```python
from build123d import *

# Parameters (mm, degrees)
SKETCH1_R           = 1.25
SKETCH1_R_2         = 1.5875
SKETCH1_R_3         = 1.587499999
SKETCH1_R_4         = 3
BOSS_EXTRUDE1_DEPTH = 3.175


with BuildPart() as part:
    # Sketch1 → Boss-Extrude1 (new body)
    with BuildSketch(Plane(origin=(0, 0, 0), x_dir=(1, 0, 0), z_dir=(0, 1, 0))):
        with BuildLine():
            Line((-19.061691445, 152.305177286), (-29.109279467, 70.814859111))
            ThreePointArc((-29.109279467, 70.814859111), (-29.106764186, 70.406916612), (-29.000369251, 70.01308476))
            Line((-29.000369251, 70.01308476), (-24.900498144, 60.115120329))
            ThreePointArc((-24.900498144, 60.115120329), (-24.059191565, 59.263489811), (-22.862282328, 59.241590515))
            ThreePointArc((-22.862282328, 59.241590515), (0, 63.5), (22.862282328, 59.241590515))
            ThreePointArc((22.862282328, 59.241590515), (24.059191565, 59.263489811), (24.900498144, 60.115120329))
            Line((24.900498144, 60.115120329), (29.000369251, 70.01308476))
            ThreePointArc((29.000369251, 70.01308476), (29.106764186, 70.406916612), (29.109279467, 70.814859111))
            Line((29.109279467, 70.814859111), (19.061691445, 152.305177286))
            ThreePointArc((19.061691445, 152.305177286), (19.052985039, 152.398309253), (19.049778848, 152.491792328))
            ThreePointArc((19.049778848, 152.491792328), (0, 171.45), (-19.049778848, 152.491792328))
            ThreePointArc((-19.049778848, 152.491792328), (-19.052985039, 152.398309253), (-19.061691445, 152.305177286))
        make_face()
        with Locations(Location((-10.606601718, 163.006601718, 0), (0, 0, 270))):
            Circle(SKETCH1_R, mode=Mode.SUBTRACT)
        with Locations(Location((0, 69.85, 0), (0, 0, 270))):
            Circle(SKETCH1_R_2, mode=Mode.SUBTRACT)
        with Locations(Location((18.0785103, 67.469918962, 0), (0, 0, 270))):
            Circle(SKETCH1_R_2, mode=Mode.SUBTRACT)
        with Locations(Location((10.606601718, 163.006601718, 0), (0, 0, 270))):
            Circle(SKETCH1_R, mode=Mode.SUBTRACT)
        with Locations(Location((10.606601718, 141.793398282, 0), (0, 0, 270))):
            Circle(SKETCH1_R, mode=Mode.SUBTRACT)
        with Locations(Location((-10.606601718, 141.793398282, 0), (0, 0, 270))):
            Circle(SKETCH1_R, mode=Mode.SUBTRACT)
        with Locations(Location((-18.078510302, 67.469918971, 0), (0, 0, 270))):
            Circle(SKETCH1_R_3, mode=Mode.SUBTRACT)
        with Locations(Location((0, 152.4, 0), (0, 0, 270))):
            Circle(SKETCH1_R_4, mode=Mode.SUBTRACT)
        with BuildLine():
            Line((-13.497810395, 120.266290898), (-4.865408959, 77.838541906))
            ThreePointArc((-4.865408959, 77.838541906), (-5.15124286, 76.569257194), (-6.289995152, 75.939949704))
            ThreePointArc((-6.289995152, 75.939949704), (-13.288948331, 75.032285399), (-20.173905346, 73.480974021))
            ThreePointArc((-20.173905346, 73.480974021), (-21.632306598, 73.810794489), (-22.169764015, 75.206092049))
            Line((-22.169764015, 75.206092049), (-16.629007128, 120.144045384))
            ThreePointArc((-16.629007128, 120.144045384), (-15.115368796, 121.53607252), (-13.497810395, 120.266290898))
        make_face(mode=Mode.SUBTRACT)
        with BuildLine():
            Line((-9.626782179, 133.089731304), (-1.555627758, 93.42047862))
            ThreePointArc((-1.555627758, 93.42047862), (0, 92.149488537), (1.555627758, 93.42047862))
            Line((1.555627758, 93.42047862), (9.626782179, 133.089731304))
            ThreePointArc((9.626782179, 133.089731304), (9.075338598, 134.635781943), (7.450296388, 134.867299588))
            ThreePointArc((7.450296388, 134.867299588), (0, 133.35), (-7.450296388, 134.867299588))
            ThreePointArc((-7.450296388, 134.867299588), (-9.075338598, 134.635781943), (-9.626782179, 133.089731304))
        make_face(mode=Mode.SUBTRACT)
        with BuildLine():
            Line((4.854451798, 161.744579859), (1.122532015, 158.012660076))
            ThreePointArc((1.122532015, 158.012660076), (0, 157.547692091), (-1.122532015, 158.012660076))
            Line((-1.122532015, 158.012660076), (-4.854451798, 161.744579859))
            ThreePointArc((-4.854451798, 161.744579859), (-5.280651093, 163.215805982), (-4.265051181, 164.36241357))
            ThreePointArc((-4.265051181, 164.36241357), (0, 165.1), (4.265051181, 164.36241357))
            ThreePointArc((4.265051181, 164.36241357), (5.280651093, 163.215805982), (4.854451798, 161.744579859))
        make_face(mode=Mode.SUBTRACT)
        with BuildLine():
            Line((-1.122532015, 146.787339924), (-4.854451798, 143.055420141))
            ThreePointArc((-4.854451798, 143.055420141), (-5.280651093, 141.584194018), (-4.265051181, 140.43758643))
            ThreePointArc((-4.265051181, 140.43758643), (0, 139.7), (4.265051181, 140.43758643))
            ThreePointArc((4.265051181, 140.43758643), (5.280651093, 141.584194018), (4.854451798, 143.055420141))
            Line((4.854451798, 143.055420141), (1.122532015, 146.787339924))
            ThreePointArc((1.122532015, 146.787339924), (0, 147.252307909), (-1.122532015, 146.787339924))
        make_face(mode=Mode.SUBTRACT)
        with BuildLine():
            Line((9.344579859, 157.254451798), (5.612660076, 153.522532015))
            ThreePointArc((5.612660076, 153.522532015), (5.147692091, 152.4), (5.612660076, 151.277467985))
            Line((5.612660076, 151.277467985), (9.344579859, 147.545548202))
            ThreePointArc((9.344579859, 147.545548202), (10.815805982, 147.119348907), (11.96241357, 148.134948819))
            ThreePointArc((11.96241357, 148.134948819), (12.7, 152.4), (11.96241357, 156.665051181))
            ThreePointArc((11.96241357, 156.665051181), (10.815805982, 157.680651093), (9.344579859, 157.254451798))
        make_face(mode=Mode.SUBTRACT)
        with BuildLine():
            Line((4.865408959, 77.838541906), (13.497810395, 120.266290898))
            ThreePointArc((13.497810395, 120.266290898), (15.115368796, 121.53607252), (16.629007128, 120.144045384))
            Line((16.629007128, 120.144045384), (22.169764015, 75.206092049))
            ThreePointArc((22.169764015, 75.206092049), (21.632306598, 73.810794489), (20.173905346, 73.480974021))
            ThreePointArc((20.173905346, 73.480974021), (13.288948331, 75.032285399), (6.289995152, 75.939949704))
            ThreePointArc((6.289995152, 75.939949704), (5.15124286, 76.569257194), (4.865408959, 77.838541906))
        make_face(mode=Mode.SUBTRACT)
        with BuildLine():
            Line((-5.612660076, 153.522532015), (-9.344579859, 157.254451798))
            ThreePointArc((-9.344579859, 157.254451798), (-10.815805982, 157.680651093), (-11.96241357, 156.665051181))
            ThreePointArc((-11.96241357, 156.665051181), (-12.7, 152.4), (-11.96241357, 148.134948819))
            ThreePointArc((-11.96241357, 148.134948819), (-10.815805982, 147.119348907), (-9.344579859, 147.545548202))
            Line((-9.344579859, 147.545548202), (-5.612660076, 151.277467985))
            ThreePointArc((-5.612660076, 151.277467985), (-5.147692091, 152.4), (-5.612660076, 153.522532015))
        make_face(mode=Mode.SUBTRACT)
    extrude(amount=BOSS_EXTRUDE1_DEPTH)


solid = part.part
```
Geometry check sheet. Reference: the model listing, model coordinates, mm. Round coordinates to 2 decimals unless told otherwise and drop trailing zeros. Order: outer loops, then holes, each group sorted by start corner. A loop starts at its lowest first (then second) coordinate and runs counter-clockwise, first axis right, second up. Notation, with made-up numbers: M 13.5,-1.5 L 69.5,-1.5 A19 cw 69.5,24.5 Z; hole C 53,41.25 d5. An arc over 180 degrees is marked long. Answer as CSV lines item,"result".
1) Mould release check, pull along Z, two halves, no side actions. Record for faces 1 (the face through (10.838, 1.565, -157.676)), 2 (the face through (6, 0, -104)): +Z half, -Z half, draft (parallel to the pull), parting line (faces both ways), or undercut.
Entries:
face 1,"undercut"
face 2,"draft"
2) Sectioned sample at B-B on z = -105.5. Record the cut outline in (x, y) (3 decimals), and give its area (3 significant figures).
Entries:
outline,"M -24.833,0 L -18.435,0 L -18.435,3.175 L -24.833,3.175 Z; M -10.493,0 L -4.013,0 L -4.013,3.175 L -10.493,3.175 Z; M 4.013,0 L 10.493,0 L 10.493,3.175 L 4.013,3.175 Z; M 18.435,0 L 24.833,0 L 24.833,3.175 L 18.435,3.175 Z"
area,"81.8 mm2"
3) Gauge pin test, flat ends, axial feed: pin 1 Ø1.5 at (y, z) = (1.5, -119.5) entering from -X; pin 2 Ø5.5 at (x, z) = (0, -152.4) entering from +Y. Record the tip position at first contact, or that the pin passes through.
Entries:
pin 1,"x = -23.2"
pin 2,"through"
4) Sectioned sample at A-A on x = 0. Give the number of separate pieces and of enclosed holes in the cut face, and give its area (3 significant figures).
Entries:
separate pieces,"6"
enclosed holes,"0"
area,"135 mm2"
5) Thickness scan on probe 1 along X at (y, z) = (1.25, -152.4); probe 2 along X at (y, z) = (1.1, -102); probe 3 along X at (y, z) = (1, -79.5). Record the ranges inside material, lowest first. Write a range as [from, to].
Entries:
probe 1,"[-19.05, -12.7], [-5.15, -3], [3, 5.15], [12.7, 19.05]"
probe 2,"[-25.26, -18.87], [-9.78, -3.3], [3.3, 9.78], [18.87, 25.26]"
probe 3,"[-28.04, -21.64], [-5.2, 5.2], [21.64, 28.04]"
